from build123d import *

# Parameters (mm, degrees)
F0_R     = 3
F1_DEPTH = 128
F2_W     = 10
F2_H     = 3.727433
F3_DEPTH = 7
F4_W     = 10
F4_H     = 10
F5_DEPTH = 7
F6_R     = 1
F7_DEPTH = 10
F8_R     = 2.5
F9_DEPTH = 110


with BuildPart() as f1:
    # F0 (on Right) → F1 (new body)
    with BuildSketch(Plane.YZ):
        Circle(F0_R)
    extrude(amount=F1_DEPTH)

    # F2 (on face) → F3 (cut)
    with BuildSketch(Plane.YZ.offset(128)):
        with Locations((0, 2.863716)):
            Rectangle(F2_W, F2_H)
    extrude(amount=-F3_DEPTH, mode=Mode.SUBTRACT)

    # F4 (on face) → F5 (cut)
    with BuildSketch(Plane.YZ.offset(128)):
        with Locations((0, -6)):
            Rectangle(F4_W, F4_H)
    extrude(amount=-F5_DEPTH, mode=Mode.SUBTRACT)

    # F6 (on face) → F7 (cut)
    with BuildSketch(Plane.XY.offset(1)):
        with Locations((125, 0)):
            Circle(F6_R)
    extrude(amount=-F7_DEPTH, mode=Mode.SUBTRACT)

    # F8 (on face) → F9 (cut)
    with BuildSketch(Plane(origin=(0, 0, 0), x_dir=(0, -1, 0), z_dir=(-1, 0, 0))):
        Circle(F8_R)
    extrude(amount=-F9_DEPTH, mode=Mode.SUBTRACT)


solid = f1.part
Geometry: final body of the model. Coordinates: model frame, mm. A direction names the side the tool comes from. Give positions to 0.01 mm unless a question says otherwise; leave off trailing zeros. Write each loop counter-clockwise with the first axis right and the second up, starting at its lowest first coordinate (ties: lowest second). Pieces come first, ordered by that corner, then holes.
(1) Access query for faces 1 (the flat face through (121, 0, -2)), 2 (the flat face through (128, 0, 0)), 3 (the flat face through (110, 0, 0)), 4 (the flat face through (123.8, 0, 1)). Directions: +Z, -Z, +X, -X, +Y, -Y. A direction counts if a zero-diameter tool reaches every point of the face in a straight line with its end or side. Return the directions, or none.
(2) Mould query, pull axis Y, two halves, no side actions, for faces 5 (the flat face through (0, -2, 2)), 6 (the cylindrical face through (54.23, 0.54, -2.44)), 7 (the cylindrical face through (63, -3, 0)). Classes: released by +Y, released by -Y, zero draft, split by the parting line, or undercut.
(3) First-contact query: P1, Ø2.5, axis at x = 125, y = 0, coming from the +Z side; P2, Ø1.5, axis at x = 80, z = -1.5, coming from the -Y side; P3, Ø2.5, axis at y = 0, z = 0.5, coming from the -X side. Flat tips, straight axial feed; report the tip coordinate or a pass-through.
(4) Cut plane C-C, the plane x = 94. Return loops of the section in (y, z).
(5) Cut plane A-A, the plane y = 0. Return loops of the section in (x, z).
(6) Cut plane B-B, the plane z = 0. Return loops of the section in (x, y).
(7) Ray query, line 1 (Z direction, x = 28, y = 0); line 2 (Y direction, x = 125, z = -0.3); line 3 (X direction, y = -1.65, z = 0). Return the intervals inside material, ascending.
Values follow:
1. face 1: -Z, +X, +Y, -Y
1. face 2: +Z, -Z, +X, +Y, -Y
1. face 3: -X
1. face 4: +Z, +X, +Y, -Y
2. face 5: zero draft
2. face 6: undercut
2. face 7: split by the parting line
3. P1: stops at z = 1
3. P2: stops at y = -2.9
3. P3: stops at x = 110
4. outline: circle Ø6 at (0, 0); hole circle Ø5 at (0, 0)
5. outline: (0, -3) - (121, -3) - (121, -1) - (124, -1) - (124, 1) - (121, 1) - (121, 3) - (0, 3) - (0, 2.5) - (110, 2.5) - (110, -2.5) - (0, -2.5) - close; (126, -1) - (128, -1) - (128, 1) - (126, 1) - close
6. outline: (0, -3) - (128, -3) - (128, 3) - (0, 3) - (0, 2.5) - (110, 2.5) - (110, -2.5) - (0, -2.5) - close; hole circle Ø2 at (125, 0)
7. line 1: z = -3 to -2.5, 2.5 to 3
7. line 2: y = -2.98 to -1, 1 to 2.98
7. line 3: x = 110 to 128
